The listing builds one solid part. Answer for the finished solid, in the listing's coordinates (mm). Face numbers are marked on the shaded views. A direction names the side the tool comes from. Give positions to 0.01 mm unless a question says otherwise; leave off trailing zeros. Loops run counter-clockwise (first coordinate to the right, second up) from the corner with the lowest first, then second, coordinate; pieces in that order, holes last. Notation, with made-up numbers: (66, 4) - (112, 4) arc R12 cw to (112, 10) - close; hole circle Ø3 at (59.5, 67.25). An arc over 180 degrees is marked (long way). One line per item, written item: value. Start each with the question number.
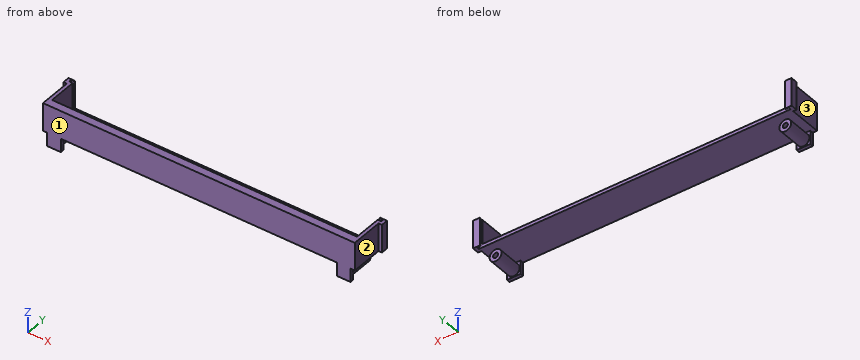
from build123d import *

# Parameters (mm, degrees)
SKIZZE1_W                        = 180
SKIZZE1_H                        = 14.5
AUFSATZ_LINEAR_AUSTRAGEN1_DEPTH  = 4.5
SCHNITT_LINEAR_AUSTRAGEN2_DEPTH  = 181.202143439
SKIZZE4_W                        = 180
SKIZZE4_H                        = 2
AUFSATZ_LINEAR_AUSTRAGEN2_DEPTH  = 21
SKIZZE5_W                        = 8
SKIZZE5_H                        = 8
AUFSATZ_LINEAR_AUSTRAGEN3_DEPTH  = 2
SKIZZE6_R                        = 3.5
AUFSATZ_LINEAR_AUSTRAGEN4_DEPTH  = 14.5
SKIZZE7_R                        = 1.5
SCHNITT_LINEAR_AUSTRAGEN3_DEPTH  = 10
SKIZZE8_W                        = 16.5
SKIZZE8_H                        = 2
AUFSATZ_LINEAR_AUSTRAGEN5_DEPTH  = 2
SKIZZE9_W                        = 2
SKIZZE9_H                        = 16.5
AUFSATZ_LINEAR_AUSTRAGEN6_DEPTH  = 2
SKIZZE10_W                       = 16.5
SKIZZE10_H                       = 0.5
AUFSATZ_LINEAR_AUSTRAGEN7_DEPTH  = 2
SKIZZE11_W                       = 16.5
SKIZZE11_H                       = 2
AUFSATZ_LINEAR_AUSTRAGEN8_DEPTH  = 2
SKIZZE12_W                       = 2
SKIZZE12_H                       = 16.5
AUFSATZ_LINEAR_AUSTRAGEN9_DEPTH  = 2
SKIZZE13_W                       = 16.5
SKIZZE13_H                       = 0.498323608
AUFSATZ_LINEAR_AUSTRAGEN10_DEPTH = 2


with BuildPart() as part:
    # Skizze1 → Aufsatz-Linear austragen1 (new body)
    with BuildSketch(Plane(origin=(0, 0, 0), x_dir=(1, 0, 0), z_dir=(0, 1, 0))):
        Rectangle(SKIZZE1_W, SKIZZE1_H)
    extrude(amount=AUFSATZ_LINEAR_AUSTRAGEN1_DEPTH)

    # Skizze2 → Schnitt-Linear austragen2 (cut, through all)
    with BuildSketch(Plane.ZY.offset(90)):
        Polygon((-7.25, 4.5), (-7.25, 1.5), (7.25, 4.5), align=None)
    extrude(amount=-SCHNITT_LINEAR_AUSTRAGEN2_DEPTH, mode=Mode.SUBTRACT)

    # Skizze4 → Aufsatz-Linear austragen2 (add)
    with BuildSketch(Plane(origin=(0, 0, 0), x_dir=(1, 0, 0), z_dir=(0, 1, 0))):
        with Locations((0, 8.25)):
            Rectangle(SKIZZE4_W, SKIZZE4_H)
        Polygon((90, 9.25), (90, 7.25), (90, -7.25), (92, -7.25), (92, 9.25), align=None)
        Polygon((-90, -7.25), (-90, 7.25), (-90, 9.25), (-92, 9.25), (-92, -7.25), align=None)
    extrude(amount=AUFSATZ_LINEAR_AUSTRAGEN2_DEPTH)

    # Skizze5 → Aufsatz-Linear austragen3 (add)
    with BuildSketch(Plane(origin=(0, 0, 0), x_dir=(1, 0, 0), z_dir=(0, 1, 0))):
        with Locations((-85.5, 13.25)):
            Rectangle(SKIZZE5_W, SKIZZE5_H)
        with Locations((85.5, 13.25)):
            Rectangle(SKIZZE5_W, SKIZZE5_H)
    extrude(amount=AUFSATZ_LINEAR_AUSTRAGEN3_DEPTH)

    # Skizze6 → Aufsatz-Linear austragen4 (add)
    with BuildSketch(Plane(origin=(0, 2, 0), x_dir=(1, 0, 0), z_dir=(0, 1, 0))):
        with Locations(Location((-85.5, 13.25, 0), (0, 0, 90))):
            Circle(SKIZZE6_R)
        with Locations(Location((85.5, 13.25, 0), (0, 0, 90))):
            Circle(SKIZZE6_R)
    extrude(amount=AUFSATZ_LINEAR_AUSTRAGEN4_DEPTH)

    # Skizze7 → Schnitt-Linear austragen3 (cut)
    with BuildSketch(Plane(origin=(0, 16.5, 0), x_dir=(1, 0, 0), z_dir=(0, 1, 0))):
        with Locations(Location((85.5, 13.25, 0), (0, 0, 270))):
            Circle(SKIZZE7_R)
        with Locations(Location((-85.5, 13.25, 0), (0, 0, 270))):
            Circle(SKIZZE7_R)
    extrude(amount=-SCHNITT_LINEAR_AUSTRAGEN3_DEPTH, mode=Mode.SUBTRACT)

    # Skizze8 → Aufsatz-Linear austragen5 (add)
    with BuildSketch(Plane(origin=(92, 0, 0), x_dir=(0, 0, -1), z_dir=(1, 0, 0))):
        with Locations((1, 20)):
            Rectangle(SKIZZE8_W, SKIZZE8_H)
    extrude(amount=AUFSATZ_LINEAR_AUSTRAGEN5_DEPTH)

    # Skizze9 → Aufsatz-Linear austragen6 (add)
    with BuildSketch(Plane(origin=(0, 21, 0), x_dir=(1, 0, 0), z_dir=(0, 1, 0))):
        with Locations((93, 1)):
            Rectangle(SKIZZE9_W, SKIZZE9_H)
    extrude(amount=AUFSATZ_LINEAR_AUSTRAGEN6_DEPTH)

    # Skizze10 → Aufsatz-Linear austragen7 (add)
    with BuildSketch(Plane.ZY.offset(-92)):
        with Locations((-1, 22.75)):
            Rectangle(SKIZZE10_W, SKIZZE10_H)
    extrude(amount=AUFSATZ_LINEAR_AUSTRAGEN7_DEPTH)

    # Skizze11 → Aufsatz-Linear austragen8 (add)
    with BuildSketch(Plane.ZY.offset(92)):
        with Locations((-1, 20)):
            Rectangle(SKIZZE11_W, SKIZZE11_H)
    extrude(amount=AUFSATZ_LINEAR_AUSTRAGEN8_DEPTH)

    # Skizze12 → Aufsatz-Linear austragen9 (add)
    with BuildSketch(Plane(origin=(0, 21, 0), x_dir=(1, 0, 0), z_dir=(0, 1, 0))):
        with Locations((-93, 1)):
            Rectangle(SKIZZE12_W, SKIZZE12_H)
    extrude(amount=AUFSATZ_LINEAR_AUSTRAGEN9_DEPTH)

    # Skizze13 → Aufsatz-Linear austragen10 (add)
    with BuildSketch(Plane(origin=(-92, 0, 0), x_dir=(0, 0, -1), z_dir=(1, 0, 0))):
        with Locations((1, 22.750838196)):
            Rectangle(SKIZZE13_W, SKIZZE13_H)
    extrude(amount=AUFSATZ_LINEAR_AUSTRAGEN10_DEPTH)


solid = part.part
1. A cutting plane is placed at C-C (z = 5.25). Determine the outline of the cut face in (x, y), plus the area to 3 significant figures.
2. Find the intervals of material crossed by L1, parallel to Z at x = -85.5, y = 12.75; L2, parallel to X at y = 13, z = -13.25; L3, parallel to X at y = 18, z = 4.5, in increasing order. Write a range as [from, to].
3. A cutting plane is placed at A-A (z = -2.5). Determine the outline of the cut face in (x, y).
4. A cutting plane is placed at B-B (x = 44.5). Determine the outline of the cut face in (y, z), plus the area to 3 significant figures.
5. For the marked faces 1, 2 and 3, determine the directions among +Z, -Z, +X, -X, +Y, -Y from which every point of the face is accessible in a straight line to the end or side of a thin tool.
6. Flat-ended cylindrical pins translate along their axes: pin 1 (4 mm diameter, centred on x = -85.5, z = -13.25, fed in from -Y); pin 2 (3 mm diameter, centred on x = 47, y = 16, fed in from -Z); pin 3 (6.5 mm diameter, centred on x = -85, z = -13.5, fed in from +Y); pin 4 (0.6 mm diameter, centred on y = 1.5, z = -12, fed in from -X). Find the tip coordinate at first contact, or state that the pin passes through.
Results below:
1. outline: (-94, 19) - (-92, 19) - (-92, 0) - (92, 0) - (92, 19) - (94, 19) - (94, 23) - (90, 23) - (90, 22.5) - (92, 22.5) - (92, 21) - (90, 21) - (90, 4.09) - (-90, 4.09) - (-90, 21) - (-92, 21) - (-92, 22.5) - (-90, 22.5) - (-90, 23) - (-94, 23) - close
1. area: 838 mm^2
2. L1: z = [-16.75, -14.75], [-11.75, -9.75], [-9.25, -7.25]
2. L2: x = [-89, -87], [-84, -82], [82, 84], [87, 89]
2. L3: x = [-92, -90], [90, 92]
3. outline: (-94, 19) - (-92, 19) - (-92, 0) - (92, 0) - (92, 19) - (94, 19) - (94, 23) - (90, 23) - (90, 22.5) - (92, 22.5) - (92, 21) - (90, 21) - (90, 2.48) - (-90, 2.48) - (-90, 21) - (-92, 21) - (-92, 22.5) - (-90, 22.5) - (-90, 23) - (-94, 23) - close
4. outline: (0, -9.25) - (21, -9.25) - (21, -7.25) - (1.5, -7.25) - (4.5, 7.25) - (0, 7.25) - close
4. area: 85.5 mm^2
5. face 1: +Z, -Z, +X, -X, -Y
5. face 2: +Z, -Z, +X, -Y
5. face 3: +Z, -Z, -X, -Y
6. pin 1: stops at y = 0
6. pin 2: stops at z = -9.25
6. pin 3: stops at y = 16.5
6. pin 4: stops at x = -89.5
